Autodesk Inventor part; units mm, degrees
ref_plane "YZ Plane" through (0, 0, 0) normal (1, 0, 0) x (0, 1, 0)
ref_plane "XZ Plane" through (0, 0, 0) normal (0, 1, 0) x (-1, 0, 0)
ref_plane "XY Plane" through (0, 0, 0) normal (0, 0, 1) x (1, 0, 0)
sketch "Sketch1" plane through (0, 0, 0) normal (0, 0, 1) x (1, 0, 0)
  circle A0 centre (0, 0) radius 28.575
  circle A1 centre (0, 0) radius 23.8125 construction
  circle A2 centre (0, 0) radius 11.1125
  line L0 (0, 0) -> (0, 28.575) construction
  circle A3 centre (0, 23.8125) radius 1.5
  line L1 (-1.5875, 10.9985) -> (-1.5875, 28.5309)
  line L2 (1.5875, 10.9985) -> (1.5875, 28.5309)
  arc A4 (7.1541, 22.7124) -> (1.5875, 18.6296) centre (5.868, 18.6296) ccw
  arc A5 (-1.5875, 18.6296) -> (-7.1541, 22.7124) centre (-5.868, 18.6296) ccw
  arc A6 (1.5875, 15.1594) -> (4.8218, 10.0119) centre (7.3009, 15.1594) ccw
  arc A7 (-4.8218, 10.0119) -> (-1.5875, 15.1594) centre (-7.3009, 15.1594) ccw
  arc A8 (-15.1594, 1.5875) -> (-10.0119, 4.8218) centre (-15.1594, 7.3009) ccw
  line L3 (-10.9985, 1.5875) -> (-28.5309, 1.5875)
  line L4 (-10.9985, -1.5875) -> (-28.5309, -1.5875)
  arc A9 (-10.0119, -4.8218) -> (-15.1594, -1.5875) centre (-15.1594, -7.3009) ccw
  arc A10 (-22.7124, 7.1541) -> (-18.6296, 1.5875) centre (-18.6296, 5.868) ccw
  arc A11 (-18.6296, -1.5875) -> (-22.7124, -7.1541) centre (-18.6296, -5.868) ccw
  circle A12 centre (-23.8125, 0) radius 1.5
  arc A13 (-1.5875, -15.1594) -> (-4.8218, -10.0119) centre (-7.3009, -15.1594) ccw
  line L5 (-1.5875, -10.9985) -> (-1.5875, -28.5309)
  line L6 (1.5875, -10.9985) -> (1.5875, -28.5309)
  arc A14 (4.8218, -10.0119) -> (1.5875, -15.1594) centre (7.3009, -15.1594) ccw
  arc A15 (-7.1541, -22.7124) -> (-1.5875, -18.6296) centre (-5.868, -18.6296) ccw
  arc A16 (1.5875, -18.6296) -> (7.1541, -22.7124) centre (5.868, -18.6296) ccw
  circle A17 centre (0, -23.8125) radius 1.5
  arc A18 (15.1594, -1.5875) -> (10.0119, -4.8218) centre (15.1594, -7.3009) ccw
  line L7 (10.9985, -1.5875) -> (28.5309, -1.5875)
  line L8 (10.9985, 1.5875) -> (28.5309, 1.5875)
  arc A19 (10.0119, 4.8218) -> (15.1594, 1.5875) centre (15.1594, 7.3009) ccw
  arc A20 (22.7124, -7.1541) -> (18.6296, -1.5875) centre (18.6296, -5.868) ccw
  arc A21 (18.6296, 1.5875) -> (22.7124, 7.1541) centre (18.6296, 5.868) ccw
  circle A22 centre (23.8125, 0) radius 1.5
  circle A23 centre (0, 0) radius 7.9375
  arc A24 (-7.1541, 22.7124) -> (-22.7124, 7.1541) centre (0, 0) ccw
  arc A25 (-23.2466, 5.1606) -> (-17.5518, -16.0925) centre (0, 0) ccw
  arc A26 (-16.0925, -17.5518) -> (5.1606, -23.2466) centre (0, 0) ccw
  arc A27 (7.1541, -22.7124) -> (22.7124, -7.1541) centre (0, 0) ccw
  arc A28 (23.2466, -5.1606) -> (17.5518, 16.0925) centre (0, 0) ccw
  arc A29 (16.0925, 17.5518) -> (-5.1606, 23.2466) centre (0, 0) ccw
  line L9 (-1.5875, 28.5309) -> (-1.5875, 31.0709)
  line L10 (-1.5875, 31.0709) -> (1.5875, 28.5309)
  line L11 (-16.9102, 26.1144) -> (-12.8906, 25.5022)
  line L12 (-15.6402, 23.9147) -> (-16.9102, 26.1144)
  line L13 (-27.7019, 14.1606) -> (-23.9147, 15.6402)
  line L14 (-25.5022, 12.8906) -> (-27.7019, 14.1606)
  line L15 (-31.0709, -1.5875) -> (-28.5309, 1.5875)
  line L16 (-28.5309, -1.5875) -> (-31.0709, -1.5875)
  line L17 (-26.1144, -16.9102) -> (-25.5022, -12.8906)
  line L18 (-23.9147, -15.6402) -> (-26.1144, -16.9102)
  line L19 (-14.1606, -27.7019) -> (-15.6402, -23.9147)
  line L20 (-12.8906, -25.5022) -> (-14.1606, -27.7019)
  line L21 (1.5875, -31.0709) -> (-1.5875, -28.5309)
  line L22 (1.5875, -28.5309) -> (1.5875, -31.0709)
  line L23 (16.9102, -26.1144) -> (12.8906, -25.5022)
  line L24 (15.6402, -23.9147) -> (16.9102, -26.1144)
  line L25 (27.7019, -14.1606) -> (23.9147, -15.6402)
  line L26 (25.5022, -12.8906) -> (27.7019, -14.1606)
  line L27 (31.0709, 1.5875) -> (28.5309, -1.5875)
  line L28 (28.5309, 1.5875) -> (31.0709, 1.5875)
  line L29 (26.1144, 16.9102) -> (25.5022, 12.8906)
  line L30 (23.9147, 15.6402) -> (26.1144, 16.9102)
  line L31 (14.1606, 27.7019) -> (15.6402, 23.9147)
  line L32 (12.8906, 25.5022) -> (14.1606, 27.7019)
  arc A30 (-22.7124, -7.1541) -> (-7.1541, -22.7124) centre (0, 0) ccw
  arc A31 (7.1541, -22.7124) -> (22.7124, -7.1541) centre (0, 0) ccw
  arc A32 (23.0011, 6.1631) -> (7.1541, 22.7124) centre (0, 0) ccw
  arc A33 (-7.1541, 22.7124) -> (-22.7124, 7.1541) centre (0, 0) ccw
  point P0 (-1.5875, 15.1594)
  point P1 (-4.8218, 10.0119)
  point P2 (-10.0119, 4.8218)
  point P3 (-1.5875, 18.6296)
  point P4 (1.5875, -15.1594)
  point P5 (4.8218, -10.0119)
  point P6 (10.0119, -4.8218)
  point P7 (-7.072, -22.7381)
  point P8 (-16.1558, -17.4936)
  point P9 (1.5875, -18.6296)
  point P10 (-28.5309, 1.5875)
  point P11 (-23.9147, -15.6402)
  point P12 (-1.5875, -28.5309)
  point P13 (1.5875, -28.5309)
  point P14 (23.9147, -15.6402)
  point P15 (25.5022, -12.8906)
  point P16 (25.5022, 12.8906)
  point P17 (23.9147, 15.6402)
  point P18 (15.1594, 1.5875)
  point P19 (7.072, -22.7381)
  point P20 (18.6296, 1.5875)
  point P21 (-15.1594, -1.5875)
  point P22 (-10.0119, -4.8218)
  point P23 (-4.8218, -10.0119)
  point P24 (-23.2278, -5.2445)
  point P25 (-22.7124, -7.1541)
  point P26 (-18.6296, -1.5875)
  point P27 (7.1541, 22.7124)
  point P28 (-23.7595, -1.5875)
  point P29 (16.0925, 17.5518)
  point P30 (17.5518, 16.0925)
  point P31 (22.7124, 7.1541)
  point P32 (-7.1541, -22.7124)
  point P33 (-16.0925, -17.5518)
  point P34 (-17.5518, -16.0925)
  point P35 (22.7124, -7.1541)
  point P36 (7.1541, -22.7124)
  dimension "d0" = 57.15
  dimension "d1" = 47.625
  dimension "d2" = 22.225
  dimension "d3" = 3
  dimension "d4" = 1.5875
  dimension "d5" = 1.5875
  dimension "d8" = 360
  dimension "d10" = 15.875
  dimension "d13" = 360
  dimension "d15" = 2.54
  dimension "d18" = 360
extrude "Extrusion1" add sketch "Sketch1" along normal blind 1 contours A0 L7 A28 A22 L8 | A0 L28 L27 | L8 A28 A32 A29 L2 A0 | A0 L6 A16 A27 A20 L7 | A0 L30 L29 | A28 A22 L7 A2 L8 | L8 A21 A28 | L26 L25 A0 | A0 L32 L31 | L8 A2 A19 | L24 L23 A0 | A18 A2 L7 | A2 | L2 A29 A3 L1 A0 | A0 L9 L10 | A2 L2 A6 | L22 L21 A0 | A0 L5 A26 A17 L6 | A14 L6 A2 | L6 A26 A17 L5 A2 | L1 A5 A24 A10 L3 A0 | A29 A4 L2 | L2 A2 L1 A29 A3 | A0 L4 A25 A30 A26 L5 | A0 L12 L11 | A2 A7 L1 | L20 L19 A0 | A26 A15 L5 | L5 A13 A2 | A0 L14 L13 | A2 L3 A8 | L18 L17 A0 | A9 L4 A2 | A2 L4 A25 A12 L3 | L3 A25 A12 L4 A0 | A0 L16 L15 | A25 L4 A11
properties part number "Wood Magnets  (UNI) V1.0." material "Titanium"
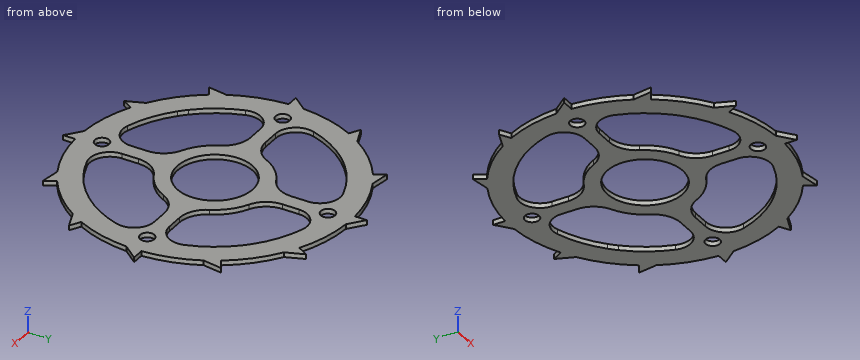
Verification items for the finished model (mm, model axes). Round coordinates to 2 decimals unless told otherwise and drop trailing zeros. Order: outer loops, then holes, each group sorted by start corner. A loop starts at its lowest first (then second) coordinate and runs counter-clockwise, first axis right, second up. Notation, with made-up numbers: (85.25, 85) -> (92.25, 85) arc R23 cw to (92.25, 115) -> close; hole circle Ø6 at (28, 11). An arc over 180 degrees is marked (long way). Put each result on its own line as item: value. Start each with the question number.
(1) Section check C-C (x = 21.5). Enter the section's corners in (y, z), then the cut area to 3 significant figures.
(2) Material ranges on line 1 along X through (y, z) = (1, 0.2); line 2 along Y through (x, z) = (-16.5, 0.55); line 3 along X through (y, z) = (-3, 0.3), recorded low to high.
(3) Depth check by flat-ended pin: pin 1 Ø0.5 at (x, z) = (30.5, 0.5) entering from +Y; pin 2 Ø2.5 at (x, y) = (23.81, 0) entering from +Z; pin 3 Ø0.5 at (y, z) = (17.5, 0.5) entering from +X. Enter the tip coordinate at first touch or a pass-through.
(4) Section check D-D (z = 0.85). State how many separate pieces and enclosed holes the cut face has, then the cut area to 3 significant figures.
(5) Section check A-A (y = 3). Enter the section's corners in (x, z).
(6) Section check B-B (x = 0). Enter the section's corners in (y, z), then the cut area to 3 significant figures.
Completed:
1. outline: (-18.82, 0) -> (-10.24, 0) -> (-10.24, 1) -> (-18.82, 1) -> close; (-2.69, 0) -> (2.69, 0) -> (2.69, 1) -> (-2.69, 1) -> close; (10.24, 0) -> (18.82, 0) -> (18.82, 1) -> (10.24, 1) -> close
1. area: 22.6 mm2
2. line 1: x = -29 to -24.93, -22.69 to -7.87, 7.87 to 22.69, 24.93 to 30.6
2. line 2: y = -23.33 to -17.17, -1.59 to 1.59, 17.17 to 23.33, 25.4 to 26.05
2. line 3: x = -28.42 to -21.81, -11.4 to -7.35, 7.35 to 11.4, 21.81 to 28.42
3. pin 1: stops at y = 1.59
3. pin 2: passes through
3. pin 3: stops at x = 22.78
4. separate pieces: 1
4. enclosed holes: 9
4. area: 1,230 mm2
5. outline: (-28.42, 0) -> (-21.81, 0) -> (-21.81, 1) -> (-28.42, 1) -> close; (-11.4, 0) -> (-7.35, 0) -> (-7.35, 1) -> (-11.4, 1) -> close; (7.35, 0) -> (11.4, 0) -> (11.4, 1) -> (7.35, 1) -> close; (21.81, 0) -> (28.42, 0) -> (28.42, 1) -> (21.81, 1) -> close
6. outline: (-29.8, 0) -> (-25.31, 0) -> (-25.31, 1) -> (-29.8, 1) -> close; (-22.31, 0) -> (-7.94, 0) -> (-7.94, 1) -> (-22.31, 1) -> close; (7.94, 0) -> (22.31, 0) -> (22.31, 1) -> (7.94, 1) -> close; (25.31, 0) -> (29.8, 0) -> (29.8, 1) -> (25.31, 1) -> close
6. area: 37.7 mm2
